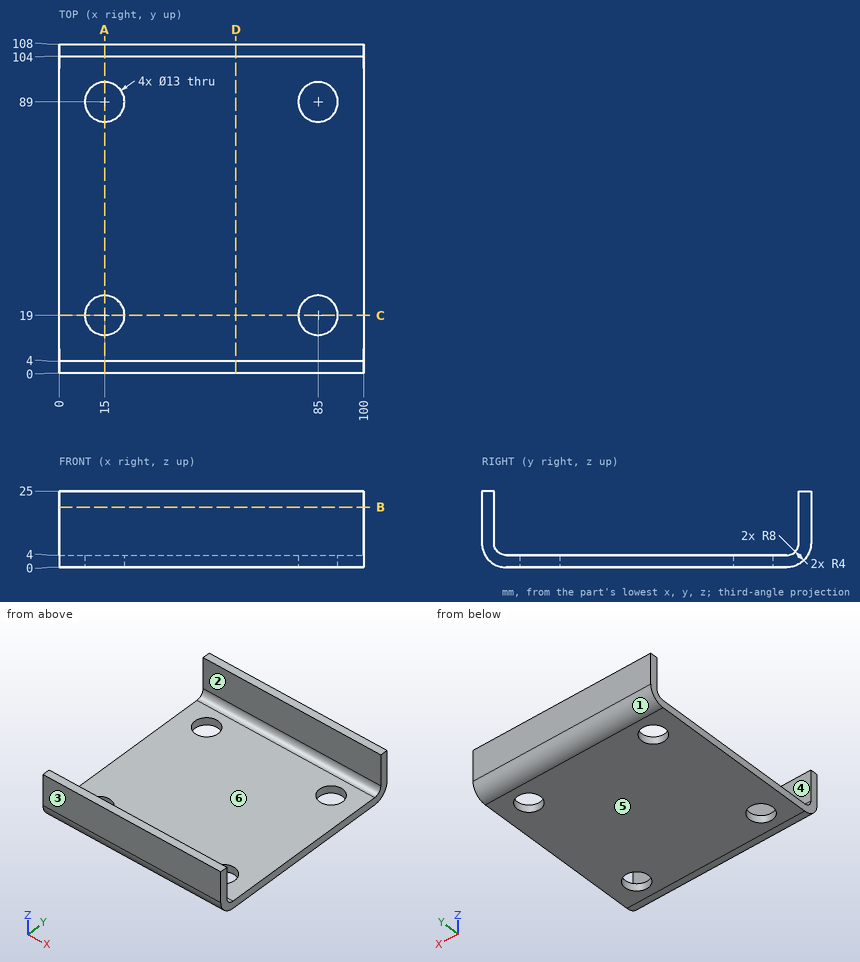
For this review, use the dimensioned drawing (mm, ordinates from the lowest corner) and the shaded views. A direction names the side the tool comes from. Give positions to 0.01 mm unless a question says otherwise; leave off trailing zeros. Order: outer loops, then holes, each group sorted by start corner. A loop starts at its lowest first (then second) coordinate and runs counter-clockwise, first axis right, second up.
1) Insertion check: pin 1 (6 mm diameter, centred on x = 17, z = 13.5, fed in from -Y); pin 2 (8 mm diameter, centred on x = 85, y = 89, fed in from -Z); pin 3 (3 mm diameter, centred on x = 36.5, y = 53, fed in from +Z). Each pin has a flat end and moves straight along its axis. Give the tip position at first contact, or say it passes through.
2) Take a section at B-B (z = 19.75). Give the boundary of the cut face in (x, y), then the cut area to 3 significant figures.
3) Take a section at D-D (x = 58). Give the boundary of the cut face in (y, z), then the cut area to 3 significant figures.
4) For the marked faces 5 and 6, list the 3-axis set-ups (+Z, -Z, +X, -X, +Y, -Y) from which the entire face can be reached by the end or side of a thin tool; tool diameter is ignored.
5) Take a section at C-C (y = 19). Give the boundary of the cut face in (x, z), then the cut area to 3 significant figures.
6) Take a section at A-A (x = 15). Give the boundary of the cut face in (y, z), then the cut area to 3 significant figures.
7) Wall thickness on line 1 (Y direction, x = 85, z = 0.95); line 2 (Y direction, x = 38, z = 19.5); line 3 (Z direction, x = 36.5, y = 26): over which ranges is each line inside the solid? List them lowest first.
8) The part is to be moulded in two halves that separate along Y. For the marked faces 1, 2, 3 and 4, say which applies: released by +Y, released by -Y, zero draft, split by the parting line, or undercut.
Derived:
1. pin 1: stops at y = 0
1. pin 2: passes through
1. pin 3: stops at z = 4
2. outline: (0, 0) - (100, 0) - (100, 4) - (0, 4) - close; (0, 104) - (100, 104) - (100, 108) - (0, 108) - close
2. area: 800 mm2
3. outline: (0, 8) arc R8 ccw to (8, 0) - (100, 0) arc R8 ccw to (108, 8) - (108, 25) - (104, 25) - (104, 8) arc R4 cw to (100, 4) - (8, 4) arc R4 cw to (4, 8) - (4, 25) - (0, 25) - close
3. area: 579 mm2
4. face 5: -Z, +X, -X, +Y, -Y
4. face 6: +Z, +X, -X
5. outline: (0, 0) - (8.5, 0) - (8.5, 4) - (0, 4) - close; (21.5, 0) - (78.5, 0) - (78.5, 4) - (21.5, 4) - close; (91.5, 0) - (100, 0) - (100, 4) - (91.5, 4) - close
5. area: 296 mm2
6. outline: (0, 8) arc R8 ccw to (8, 0) - (12.5, 0) - (12.5, 4) - (8, 4) arc R4 cw to (4, 8) - (4, 25) - (0, 25) - close; (25.5, 0) - (82.5, 0) - (82.5, 4) - (25.5, 4) - close; (95.5, 0) - (100, 0) arc R8 ccw to (108, 8) - (108, 25) - (104, 25) - (104, 8) arc R4 cw to (100, 4) - (95.5, 4) - close
6. area: 475 mm2
7. line 1: y = 4.22 to 12.5, 25.5 to 82.5, 95.5 to 103.78
7. line 2: y = 0 to 4, 104 to 108
7. line 3: z = 0 to 4
8. face 1: released by +Y
8. face 2: undercut
8. face 3: released by -Y
8. face 4: undercut
